Could you check a few things on this model? Use its own coordinates, in mm. A direction names the side the tool comes from. Give positions to 0.01 mm unless a question says otherwise; leave off trailing zeros. Loops run counter-clockwise (first coordinate to the right, second up) from the corner with the lowest first, then second, coordinate; pieces in that order, holes last. Notation, with made-up numbers: (39, 65.5) - (87, 65.5) arc R31 cw to (87, 94.5) - close; hole circle Ø11 at (-38, -39.75). An arc over 180 degrees is marked (long way). Write each question's results on one line, items separated by ' | '. Start each with the question number.
1) I want a section at B-B, the plane z = 1.35. Write out the boundary of the cut face in (x, y) (3 decimals), and give its area (3 significant figures).
2) I want a section at A-A, the plane x = 25.4. Write out the boundary of the cut face in (y, z) (3 decimals), and give its area (3 significant figures).
3) I want a section at C-C, the plane x = 47.5. Write out the boundary of the cut face in (y, z) (3 decimals).
4) If I drill on probe 1 along Y at (x, z) = (25.4, 2.4) (3 decimals); probe 2 along Y at (x, z) = (43, 0.5) (3 decimals); probe 3 along X at (y, z) = (28, 0.8), over which ranges is the centre line in solid material (lowest first)? Write a range as [from, to].
5) On a 3-axis mill with a long thin cutter (end or side, diameter ignored), from which of +Z, -Z, +X, -X, +Y, -Y can I reach the whole of each face in a straight line? I mean faces 5 (the face through (13, 9.525, 2)), 6 (the face through (2.291, 61.327, 1.565)). Say none if no direction works.
6) If we mould it in two halves opening along Y, with no side actions, what happens to faces 1 (the face through (25, 46.3, 3.175)), 2 (the face through (38, 9.525, 2)), 3 (the face through (19.05, 8, 2)), 4 (the face through (26, 63.5, 2))? For each: +Y half, -Y half, draft (parallel to the pull), parting line (faces both ways), or undercut.
from build123d import *

# Parameters (mm, degrees)
SKETCH1_R           = 17.5
SKETCH1_W           = 12.7
SKETCH1_H           = 3.175
BOSS_EXTRUDE1_DEPTH = 3.175


with BuildPart() as part:
    # Sketch1 → Boss-Extrude1 (new body)
    with BuildSketch(Plane.XY):
        with BuildLine():
            Line((0, 0), (50.8, 0))
            Line((50.8, 0), (50.8, 55.88))
            ThreePointArc((50.8, 55.88), (48.568153673, 61.268153673), (43.18, 63.5))
            Line((43.18, 63.5), (7.62, 63.5))
            ThreePointArc((7.62, 63.5), (2.231846327, 61.268153673), (0, 55.88))
            Line((0, 55.88), (0, 0))
        make_face()
        with Locations((25.4, 28.575)):
            Circle(SKETCH1_R, mode=Mode.SUBTRACT)
        with Locations((12.7, 7.9375)):
            Rectangle(SKETCH1_W, SKETCH1_H, mode=Mode.SUBTRACT)
        with Locations((38.1, 7.9375)):
            Rectangle(SKETCH1_W, SKETCH1_H, mode=Mode.SUBTRACT)
    extrude(amount=BOSS_EXTRUDE1_DEPTH)


solid = part.part
Answers:
1) outline: (0, 0) - (50.8, 0) - (50.8, 55.88) arc R7.62 ccw to (43.18, 63.5) - (7.62, 63.5) arc R7.62 ccw to (0, 55.88) - close; hole (6.35, 6.35) - (19.05, 6.35) - (19.05, 9.525) - (6.35, 9.525) - close; hole circle Ø35 at (25.4, 28.575); hole (31.75, 6.35) - (44.45, 6.35) - (44.45, 9.525) - (31.75, 9.525) - close | area: 2,160 mm2
2) outline: (0, 0) - (11.075, 0) - (11.075, 3.175) - (0, 3.175) - close; (46.075, 0) - (63.5, 0) - (63.5, 3.175) - (46.075, 3.175) - close | area: 90.5 mm2
3) outline: (0, 0) - (62.157, 0) - (62.157, 3.175) - (0, 3.175) - close
4) probe 1: y = [0, 11.075], [46.075, 63.5] | probe 2: y = [0, 6.35], [9.525, 63.5] | probe 3: x = [0, 7.91], [42.89, 50.8]
5) face 5: +Z, -Z | face 6: +Z, -Z, -X, +Y
6) face 1: draft | face 2: undercut | face 3: undercut | face 4: +Y half
